from build123d import *

# Parameters (mm, degrees)
F0_W     = 27
F0_H     = 2
F2_SIZE  = 0.2
F3_R     = 0.5
F4_DEPTH = 2.5


with BuildPart() as f1:
    # F0 (on Front) → F1 (revolve)
    with BuildSketch(Plane.XZ):
        with Locations((13.5, 1)):
            Rectangle(F0_W, F0_H)
    revolve(axis=Axis((13.5, 0, 0), (-1, 0, 0)))

    # F2
    f2_edges = [f1.edges().sort_by_distance(p)[0] for p in [
        (0, 0, -2),
        (27, 0, -2),
    ]]
    chamfer(f2_edges, length=F2_SIZE)

    # F3 (on Top) → F4 (cut, symmetric)
    with BuildSketch(Plane.XY):
        with Locations((1.7, 0)):
            Circle(F3_R)
        with Locations((25.3, 0)):
            Circle(F3_R)
    extrude(amount=F4_DEPTH, both=True, mode=Mode.SUBTRACT)


solid = f1.part
Design review of the part built by this model. Coordinates are the model's own, in mm. Round coordinates to 2 decimals unless told otherwise and drop trailing zeros. Order: outer loops, then holes, each group sorted by start corner. A loop starts at its lowest first (then second) coordinate and runs counter-clockwise, first axis right, second up.
1) Draft analysis for pull direction X (two halves, no side actions). For faces 1 (the flat face through (27, 0, 0)), 2 (the flat face through (0, 0, 0)), 3 (the cylindrical face through (25.777, 0.15, 0.027)), state which applies: released by +X, released by -X, zero draft, split by the parting line, or undercut.
The answers:
face 1: released by +X
face 2: released by -X
face 3: undercut
2) Clearance check with a flat-ended pin moving along its axis: pin 1 Ø1 at (x, y) = (4, 1) entering from -Z. State where the tip first meets the part, or that it passes through.
The answers:
pin 1: stops at z = -1.94
3) Consider section A-A (y = 0). State the section outline as (x, z) points, plus the area to 3 significant figures.
The answers:
outline: (0, -1.8) - (0.2, -2) - (1.2, -2) - (1.2, 2) - (0.2, 2) - (0, 1.8) - close; (2.2, -2) - (24.8, -2) - (24.8, 2) - (2.2, 2) - close; (25.8, -2) - (26.8, -2) - (27, -1.8) - (27, 1.8) - (26.8, 2) - (25.8, 2) - close
area: 99.9 mm2
4) Consider section B-B (x = 10.75). State the section outline as (y, z) points.
The answers:
outline: circle Ø4 at (0, 0)
5) For L1, parallel to X at y = 0, z = 0.85; L2, parallel to Y at x = 25.3, z = -0.9; L3, parallel to Y at x = 1.7, z = 1.05, list the stretches that pass through material, from the lowest coordinate up.
The answers:
L1: x = 0 to 1.2, 2.2 to 24.8, 25.8 to 27
L2: y = -1.79 to -0.5, 0.5 to 1.79
L3: y = -1.7 to -0.5, 0.5 to 1.7
6) Consider section C-C (x = 25.3). State the section outline as (y, z) points.
The answers:
outline: (-0.5, -1.94) - (-0.5, 1.94) arc R2 ccw to start; (0.5, -1.94) arc R2 ccw to (0.5, 1.94) - close
